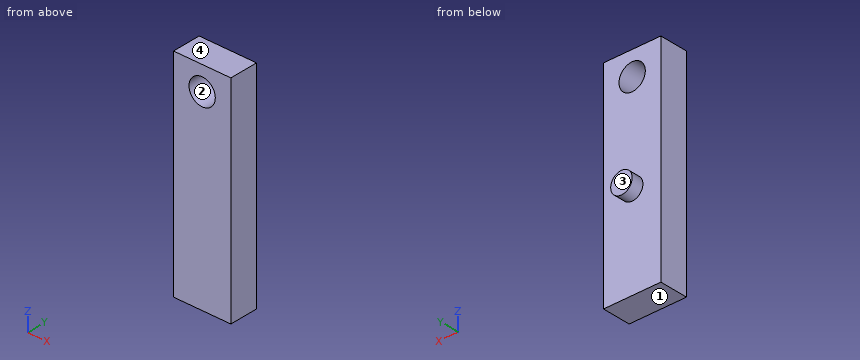
Autodesk Inventor part; units mm, degrees
ref_plane "YZ Plane" through (0, 0, 0) normal (1, 0, 0) x (0, 1, 0)
ref_plane "XZ Plane" through (0, 0, 0) normal (0, 1, 0) x (-1, 0, 0)
ref_plane "XY Plane" through (0, 0, 0) normal (0, 0, 1) x (1, 0, 0)
sketch "Sketch1" plane through (0, 0, 0) normal (0, 1, 0) x (-1, 0, 0)
  line L0 (0, 0) -> (12, 0)
  line L1 (12, 0) -> (12, -45)
  line L2 (12, -45) -> (0, -45)
  line L3 (0, -45) -> (0, 0)
  dimension "d0" = 12
  dimension "d1" = 45
extrude "Extrusion1" add sketch "Sketch1" along normal blind 6
sketch "Sketch2" plane through (0, 6, 0) normal (0, 1, 0) x (1, 0, 0)
  line L0 (-12, 0) -> (0, 0)
  line L1 (-6, 0) -> (-6, 5)
  circle A0 centre (-6, 5) radius 2.75
  dimension "d4" = 5
  dimension "d5" = 5.5
extrude "Extrusion2" cut sketch "Sketch2" against normal blind 6
sketch "Sketch3" plane through (0, 6, 0) normal (0, 1, 0) x (1, 0, 0)
  circle A0 centre (-6, 5) radius 2.75
  line L0 (-6, 5) -> (-6, 25.5)
  circle A1 centre (-6, 25.5) radius 2.25
  point P0 (0, 0)
  dimension "d8" = 20.5
  dimension "d9" = 4.5
extrude "Extrusion3" add sketch "Sketch3" along normal blind 2.5 contours A1
properties part number "limit_switch_upper_mount"
Build history of the part. All positions in model axes, mm. Face numbers are marked on the shaded views. Round coordinates to 2 decimals unless told otherwise and drop trailing zeros. Write each loop counter-clockwise with the first axis right and the second up, starting at its lowest first coordinate (ties: lowest second). Pieces come first, ordered by that corner, then holes. Notation, with made-up numbers: M 74.25,10.5 L 106.25,10.5 A17 cw 106.25,38.5 Z; hole C 64,78 d9. An arc over 180 degrees is marked long. Answer in a Markdown table with one row per item.
1. Saw through at B-B (y = 3.5). List the corners of the cut face in (x, z), and give its area (3 significant figures).
Geometry check:
| item | result |
|---|---|
| outline | M -12,-45 L 0,-45 L 0,0 L -12,0 Z; hole C -6,-5 d5.5 |
| area | 516 mm2 |
2. Mould opens along Z. For the marked faces 1, 2, 3 and 4 say: +Z half, -Z half, draft (parallel to the pull), parting line (faces both ways), or undercut.
Geometry check:
| item | result |
|---|---|
| face 1 | -Z half |
| face 2 | undercut |
| face 3 | draft |
| face 4 | +Z half |
3. Saw through at C-C (z = -5). List the corners of the cut face in (x, y).
Geometry check:
| item | result |
|---|---|
| outline | M -12,0 L -8.75,0 L -8.75,6 L -12,6 Z; M -3.25,0 L 0,0 L 0,6 L -3.25,6 Z |
4. Probe L1, parallel to X at y = 3.9, z = -5; L2, parallel to Z at x = -6, y = 1.6; L3, parallel to Y at x = -3.5, z = -22. List the from-to ranges inside material, lowest first. Write a range as [from, to].
Geometry check:
| item | result |
|---|---|
| L1 | [-12, -8.75], [-3.25, 0] |
| L2 | [-45, -7.75], [-2.25, 0] |
| L3 | [0, 6] |
5. Saw through at D-D (z = -25.5). List the corners of the cut face in (x, y).
Geometry check:
| item | result |
|---|---|
| outline | M -12,0 L 0,0 L 0,6 L -3.75,6 L -3.75,8.5 L -8.25,8.5 L -8.25,6 L -12,6 Z |
6. Saw through at A-A (x = -6). List the corners of the cut face in (y, z), and give its area (3 significant figures).
Geometry check:
| item | result |
|---|---|
| outline | M 0,-45 L 6,-45 L 6,-27.75 L 8.5,-27.75 L 8.5,-23.25 L 6,-23.25 L 6,-7.75 L 0,-7.75 Z; M 0,-2.25 L 6,-2.25 L 6,0 L 0,0 Z |
| area | 248 mm2 |
7. Flat gauge pins, fed straight in: P1, Ø6, axis at x = -7.5, z = -27, coming from the -Y side; P2, Ø1.5, axis at x = -9, z = -29.5, coming from the +Y side. Where does each tip first touch, or does it go through?
Geometry check:
| item | result |
|---|---|
| P1 | y = 0 |
| P2 | y = 6 |
